Source: CAD feature listing. Evaluate the final solid. Frame: model axes, mm. Face numbers are marked on the shaded views. A direction names the side the tool comes from. Give positions to 0.01 mm unless a question says otherwise; leave off trailing zeros. Loops run counter-clockwise (first coordinate to the right, second up) from the corner with the lowest first, then second, coordinate; pieces in that order, holes last. Notation, with made-up numbers: M 80.25,-34 L 88.25,-34 A35 cw 88.25,-2 Z; hole C 28.5,22.25 d1. An arc over 180 degrees is marked long. Answer in a Markdown table with one row per item.
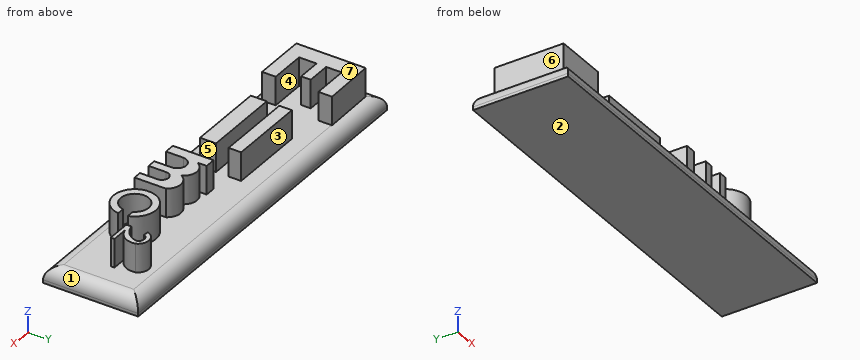
```python
from build123d import *

# Parameters (mm, degrees)
F0_W      = 152.4
F0_H      = 38.1
F1_DEPTH  = 6.35
F2_R      = 5.08
F4_DEPTH  = 11.43
F5_W      = 31.0896
F5_H      = 5.0292
F5_H_2    = 6.400801
F6_DEPTH  = 11.43
F8_DEPTH  = 11.43
F10_DEPTH = 11.43
F12_DEPTH = 11.43


with BuildPart() as f1:
    # F0 (on Top) → F1 (new body)
    with BuildSketch(Plane.XY):
        with Locations((-0.578179, -2.4384)):
            Rectangle(F0_W, F0_H)
    extrude(amount=F1_DEPTH)

    # F2
    f2_edges = [f1.edges().sort_by_distance(p)[0] for p in [
        (-0.578179, 16.6116, 6.35),
        (-76.778179, -2.4384, 6.35),
        (-0.578179, -21.4884, 6.35),
        (75.621821, -2.4384, 6.35),
    ]]
    fillet(f2_edges, radius=F2_R)

    # F3 (on face) → F4 (join)
    with BuildSketch(Plane.XY.offset(6.35)):
        Polygon((-50.58109, 11.734799), (-71.612291, 11.430001), (-71.612291, -16.306801), (-50.58109, -16.306801), (-50.58109, -10.8204), (-64.906694, -10.8204), (-64.906694, -3.81), (-55.45789, -3.81), (-55.45789, 0), (-64.906694, 0), (-64.906694, 6.2484), (-50.58109, 6.2484), align=None)
    extrude(amount=F4_DEPTH)

    # F5 (on face) → F6 (join)
    with BuildSketch(Plane.XY.offset(6.35)):
        with Locations((-20.71069, 2.5146)):
            Rectangle(F5_W, F5_H)
        with Locations((-20.71069, -8.229601)):
            Rectangle(F5_W, F5_H_2)
    extrude(amount=F6_DEPTH)

    # F7 (on face) → F8 (join)
    with BuildSketch(Plane.XY.offset(6.35)):
        with BuildLine():
            Line((3.987037, -0.034714), (3.987037, -16.323045))
            Line((3.987037, -16.323045), (8.195101, -16.323045))
            Line((8.195101, -16.323045), (8.195101, -9.309177))
            ThreePointArc((8.195101, -9.309177), (11.782139, -5.880751), (15.369177, -9.309177))
            Line((15.369177, -9.309177), (15.369177, -16.338116))
            Line((15.369177, -16.338116), (18.81415, -16.338116))
            Line((18.81415, -16.338116), (18.81415, -9.309177))
            ThreePointArc((18.81415, -9.309177), (21.455294, -6.668033), (24.096439, -9.309177))
            Line((24.096439, -9.309177), (24.096439, -16.345294))
            Line((24.096439, -16.345294), (27.413206, -16.345294))
            Line((27.413206, -16.345294), (27.413206, -3.832139))
            ThreePointArc((27.413206, -3.832139), (22.598146, -1.020168), (17.783085, -3.832139))
            ThreePointArc((17.783085, -3.832139), (12.989093, -0.790731), (8.195101, -3.832139))
            Line((8.195101, -3.832139), (8.195101, -0.034714))
            Line((8.195101, -0.034714), (3.987037, -0.034714))
        make_face()
    extrude(amount=F8_DEPTH)

    # F9 (on face) → F10 (join)
    with BuildSketch(Plane.XY.offset(6.35)):
        with BuildLine():
            Line((45.470758, -5.2382), (48.550447, -5.2382))
            ThreePointArc((48.550447, -5.2382), (32.01016, -8.446661), (48.853159, -8.881086))
            Line((48.853159, -8.881086), (45.94597, -8.881086))
            ThreePointArc((45.94597, -8.881086), (34.895535, -8.47017), (45.470758, -5.2382))
        make_face()
    extrude(amount=F10_DEPTH)

    # F11 (on face) → F12 (join)
    with BuildSketch(Plane.XY.offset(6.35)):
        with BuildLine():
            ThreePointArc((55.785455, -1.235234), (60.317074, 1.178317), (61.454367, 6.185049))
            ThreePointArc((61.454367, 6.185049), (57.275841, 8.987166), (53.296663, 5.908517))
            Line((53.296663, 5.908517), (55.232391, 5.678073))
            ThreePointArc((55.232391, 5.678073), (57.536826, 7.236442), (59.84126, 5.678073))
            ThreePointArc((59.84126, 5.678073), (57.618597, 1.433053), (53.296663, -0.63608))
            Line((53.296663, -0.63608), (53.296663, -2.710072))
            Line((53.296663, -2.710072), (62.837027, -2.710072))
            Line((62.837027, -2.710072), (62.837027, -1.235234))
            Line((62.837027, -1.235234), (55.785455, -1.235234))
        make_face()
    extrude(amount=F12_DEPTH)


solid = f1.part
```
1) Set-up query: the marked faces 4, 5, 6 and 7. Return all of +Z, -Z, +X, -X, +Y, -Y with unobstructed straight access to the full face (end or side cutting, diameter ignored); none if empty.
Reply:
| item | result |
|---|---|
| face 4 | +Z |
| face 5 | +Z, +Y, -Y |
| face 6 | +Z, -X, +Y, -Y |
| face 7 | +Z, +X, -X, +Y, -Y |
2) Material intervals for L1, parallel to Y at x = -30, z = 16; L2, parallel to X at y = -15.5, z = 12.5; L3, parallel to X at y = -15, z = 8.5, sorted ascending.
Reply:
| item | result |
|---|---|
| L1 | y = -11.43 to -5.03, 0 to 5.03 |
| L2 | x = -71.61 to -50.58, 3.99 to 8.2, 15.37 to 18.81, 24.1 to 27.41, 37.04 to 43.87 |
| L3 | x = -71.61 to -50.58, 3.99 to 8.2, 15.37 to 18.81, 24.1 to 27.41, 36.08 to 44.83 |
3) Pull-direction query (X, two-part tool) for the marked faces 1, 2 and 3; classes: released by +X, released by -X, zero draft, split by the parting line, or undercut.
Reply:
| item | result |
|---|---|
| face 1 | released by +X |
| face 2 | zero draft |
| face 3 | undercut |
4) Section C-C, the plane z = 3.75. Return loops of the section in (x, y).
Reply:
| item | result |
|---|---|
| outline | M -76.13,-20.84 L 74.98,-20.84 L 74.98,15.97 L -76.13,15.97 Z |
5) Section A-A, the plane z = 15.25. Count the separate pieces of the cut face and the enclosed holes in it, then the cut area to 3 significant figures.
Reply:
| item | result |
|---|---|
| separate pieces | 6 |
| enclosed holes | 0 |
| area | 1,130 mm² |
6) Section B-B, the plane y = 2. Return loops of the section in (x, z).
Reply:
| item | result |
|---|---|
| outline | M -76.78,0 L 75.62,0 L 75.62,1.27 A5.08 ccw 70.54,6.35 L 60.85,6.35 L 60.85,17.78 L 58.15,17.78 L 58.15,6.35 L -5.17,6.35 L -5.17,17.78 L -36.26,17.78 L -36.26,6.35 L -64.91,6.35 L -64.91,17.78 L -71.61,17.78 L -71.61,6.35 L -71.7,6.35 A5.08 ccw -76.78,1.27 Z |
7) Pin query (flat end, axial travel): pin 1 Ø1.6 at (y, z) = (-14.5, 10.5) entering from +X; pin 2 Ø6 at (y, z) = (1, 13.5) entering from -X; pin 3 Ø1 at (x, z) = (16.5, 12) entering from -Y. Return the tip coordinate at first contact, or that it passes through.
Reply:
| item | result |
|---|---|
| pin 1 | stops at x = 46.48 |
| pin 2 | stops at x = -71.61 |
| pin 3 | stops at y = -16.34 |
